from build123d import *

# Parameters (mm, degrees)
EXTRUDE_THIN1_DEPTH = 222.25
FILLET1_R           = 1.9812


with BuildPart() as part:
    # Sketch1 → Extrude-Thin1 (new body)
    with BuildSketch(Plane.XY):
        with BuildLine():
            Line((2.1844, 0), (11.1125, 0))
            Line((11.1125, 0), (11.1125, 8.73125))
            ThreePointArc((11.1125, 8.73125), (6.838482158, 11.13965279), (5.55625, 15.875))
            Line((5.55625, 15.875), (-5.55625, 15.875))
            ThreePointArc((-5.55625, 15.875), (-6.838482158, 11.13965279), (-11.1125, 8.73125))
            Line((-11.1125, 8.73125), (-11.1125, 0))
            Line((-11.1125, 0), (-2.1844, 0))
            Line((-2.1844, 0), (-2.1844, 1.9812))
            Line((-2.1844, 1.9812), (-9.1313, 1.9812))
            Line((-9.1313, 1.9812), (-9.1313, 7.163352557))
            ThreePointArc((-9.1313, 7.163352557), (-5.415045416, 9.747705801), (-3.598638875, 13.8938))
            Line((-3.598638875, 13.8938), (3.598638875, 13.8938))
            ThreePointArc((3.598638875, 13.8938), (5.415045416, 9.747705801), (9.1313, 7.163352557))
            Line((9.1313, 7.163352557), (9.1313, 1.9812))
            Line((9.1313, 1.9812), (2.1844, 1.9812))
            Line((2.1844, 1.9812), (2.1844, 0))
        make_face()
    extrude(amount=-EXTRUDE_THIN1_DEPTH)

    # Fillet1
    fillet1_edges = [part.edges().sort_by_distance(p)[0] for p in [
        (-11.1125, 0, -111.125),
        (-11.1125, 8.73125, -111.125),
        (-5.55625, 15.875, -111.125),
        (5.55625, 15.875, -111.125),
        (11.1125, 8.73125, -111.125),
        (11.1125, 0, -111.125),
    ]]
    fillet(fillet1_edges, radius=FILLET1_R)


solid = part.part
Read the model definition and answer for the solid it produces. Units are mm, in the model's axes. A direction names the side the tool comes from. Round coordinates to 2 decimals unless told otherwise and drop trailing zeros. Write each loop counter-clockwise with the first axis right and the second up, starting at its lowest first coordinate (ties: lowest second). Pieces come first, ordered by that corner, then holes.
1. Straight lines are drawn through the part: L1, parallel to X at y = 6.5, z = -207.5; L2, parallel to Y at x = 5.25, z = -149; L3, parallel to X at y = 13.25, z = -212.5. For each, find the intervals that lie inside material, in ascending order.
2. The part is cut by section C-C, the plane y = 4. Determine the outline of the cut face in (x, z), then the cut area to 3 significant figures.
3. Determine the mould class of faces 3 (the face through (6, 0, -110)), 4 (the face through (-11.112, 5, -110)), 5 (the face through (-9.131, 5, -110)), 6 (the face through (6.977, 10.968, -109.569)) for opening direction Y: pulls with the +Y half, pulls with the -Y half, needs draft (parallel to the pull), parting line crosses it, or undercut.
4. The part is cut by section A-A, the plane y = 12. Determine the outline of the cut face in (x, z).
5. Given pin 1 Ø1 at (y, z) = (0.5, -66.5) entering from +X; pin 2 Ø6 at (x, z) = (0, -80) entering from -Y; pin 3 Ø1.5 at (y, z) = (11, -134) entering from +X; pin 4 Ø1 at (y, z) = (11, -51.5) entering from +X, each flat-ended and moving along its own axis, determine where each tip first touches the part or whether it passes through.
6. Which of the six approach directions +Z, -Z, +X, -X, +Y, -Y give full straight-line access (tool end or side, diameter ignored) to faces 1 (the face through (0, 13.894, -110)), 2 (the face through (-6, 0, -110))?
Values:
1. L1: x = -11.11 to -9.13, 9.13 to 11.11
1. L2: y = 0 to 1.98, 9.96 to 14.99
1. L3: x = -5.76 to -3.71, 3.71 to 5.76
2. outline: (-11.11, -222.25) - (-9.13, -222.25) - (-9.13, 0) - (-11.11, 0) - close; (9.13, -222.25) - (11.11, -222.25) - (11.11, 0) - (9.13, 0) - close
2. area: 881 mm2
3. face 3: pulls with the -Y half
3. face 4: needs draft
3. face 5: undercut
3. face 6: pulls with the +Y half
4. outline: (-6.27, -222.25) - (-4.09, -222.25) - (-4.09, 0) - (-6.27, 0) - close; (4.09, -222.25) - (6.27, -222.25) - (6.27, 0) - (4.09, 0) - close
5. pin 1: stops at x = 10.85
5. pin 2: stops at y = 0
5. pin 3: stops at x = 7.68
5. pin 4: stops at x = 7.41
6. face 1: +Z, -Z
6. face 2: +Z, -Z, +X, -X, -Y
